from build123d import *

# Parameters (mm, degrees)
CUT_EXTRUDE3_DEPTH      = 107.301458127
CUT_EXTRUDE3_DEPTH_BACK = 107.301458127
SKETCH4_R               = 6


with BuildPart() as part:
    # Sketch1 → Revolve2 (revolve)
    with BuildSketch(Plane(origin=(0, 0, 0), x_dir=(1, 0, 0), z_dir=(0, 1, 0)), mode=Mode.PRIVATE) as revolve2_sk:
        Polygon((0, 25), (0, 40), (-19.12049302, 40), (-29.12049302, 30), (-29.12049302, 0), (0, 0), (90, 0), (90, 15), (80, 25), align=None)
    revolve(revolve2_sk.sketch.rotate(Axis((0, 0, 0), (1, 0, 0)), 180), axis=Axis((0, 0, 0), (1, 0, 0)))

    # Sketch4 → Cut-Extrude3 (cut, two sides: drawn at the far end of the back side and taken through both)
    with BuildSketch(Plane(origin=(0, 0, 0), x_dir=(1, 0, 0), z_dir=(0, 1, 0)).offset(-CUT_EXTRUDE3_DEPTH_BACK)):
        with Locations(Location((72, 0, 0), (0, 0, 270))):
            Circle(SKETCH4_R)
    extrude(amount=CUT_EXTRUDE3_DEPTH + CUT_EXTRUDE3_DEPTH_BACK, mode=Mode.SUBTRACT)


solid = part.part
Verification items for the finished model (mm, model axes). A direction names the side the tool comes from. Give positions to 0.01 mm unless a question says otherwise; leave off trailing zeros. Loops run counter-clockwise (first coordinate to the right, second up) from the corner with the lowest first, then second, coordinate; pieces in that order, holes last.
1) Depth check by flat-ended pin: pin 1 Ø4 at (x, z) = (58.5, -3) entering from +Y; pin 2 Ø6 at (x, y) = (46.5, 13) entering from +Z; pin 3 Ø5 at (x, z) = (4.5, -29.5) entering from -Y; pin 4 Ø3 at (x, z) = (50, 18) entering from +Y. Enter the tip coordinate at first touch or a pass-through.
2) Set-up check for faces 4 (the flat face through (90, 0, 0)), 5 (the cylindrical face through (39.4, 22.2, 11.5)): record each of +Z, -Z, +X, -X, +Y, -Y from which the full face is reachable in a straight line by a thin tool's end or side.
3) Sectioned sample at D-D, the plane x = 72. Enter the section's corners in (y, z).
4) Sectioned sample at B-B, the plane z = 0. Enter the section's corners in (x, y), then the cut area to 3 significant figures.
5) Thickness scan on line 1 along X through (y, z) = (-10, 0); line 2 along X through (y, z) = (-18.5, -18); line 3 along X through (y, z) = (-29, -18). Record the ranges inside material, lowest first.
6) Sectioned sample at A-A, the plane y = 0. Enter the section's corners in (x, z).
7) Sectioned sample at C-C, the plane x = 13.5. Enter the section's corners in (y, z).
8) Draft check along Z on faces 1 (the cylindrical face through (77.059, -0.35, 3.226)), 2 (the flat face through (-29.12, 0, 0)), 3 (the cylindrical face through (-9.69, -1.76, -39.96)). Enter one of: pulls with the +Z half, pulls with the -Z half, needs draft (parallel to the pull), parting line crosses it, or undercut.
Answers:
1. pin 1: stops at y = 24.98
1. pin 2: stops at z = 22.91
1. pin 3: passes through
1. pin 4: stops at y = 18.78
2. face 4: +Z, -Z, +X, +Y, -Y
2. face 5: +X
3. outline: (-24.27, -6) arc R25 ccw to (24.27, -6) - close; (-24.27, 6) - (24.27, 6) arc R25 ccw to start
4. outline: (-29.12, -30) - (-19.12, -40) - (0, -40) - (0, -25) - (66, -25) - (66, 25) - (0, 25) - (0, 40) - (-19.12, 40) - (-29.12, 30) - close; (78, -25) - (80, -25) - (90, -15) - (90, 15) - (80, 25) - (78, 25) - close
4. area: 6,030 mm2
5. line 1: x = -29.12 to 66, 78 to 90
5. line 2: x = -29.12 to 0
5. line 3: x = -24.99 to 0
6. outline: (-29.12, -30) - (-19.12, -40) - (0, -40) - (0, -25) - (80, -25) - (90, -15) - (90, 15) - (80, 25) - (0, 25) - (0, 40) - (-19.12, 40) - (-29.12, 30) - close; hole circle Ø12 at (72, 0)
7. outline: circle Ø50 at (0, 0)
8. face 1: undercut
8. face 2: needs draft
8. face 3: parting line crosses it
